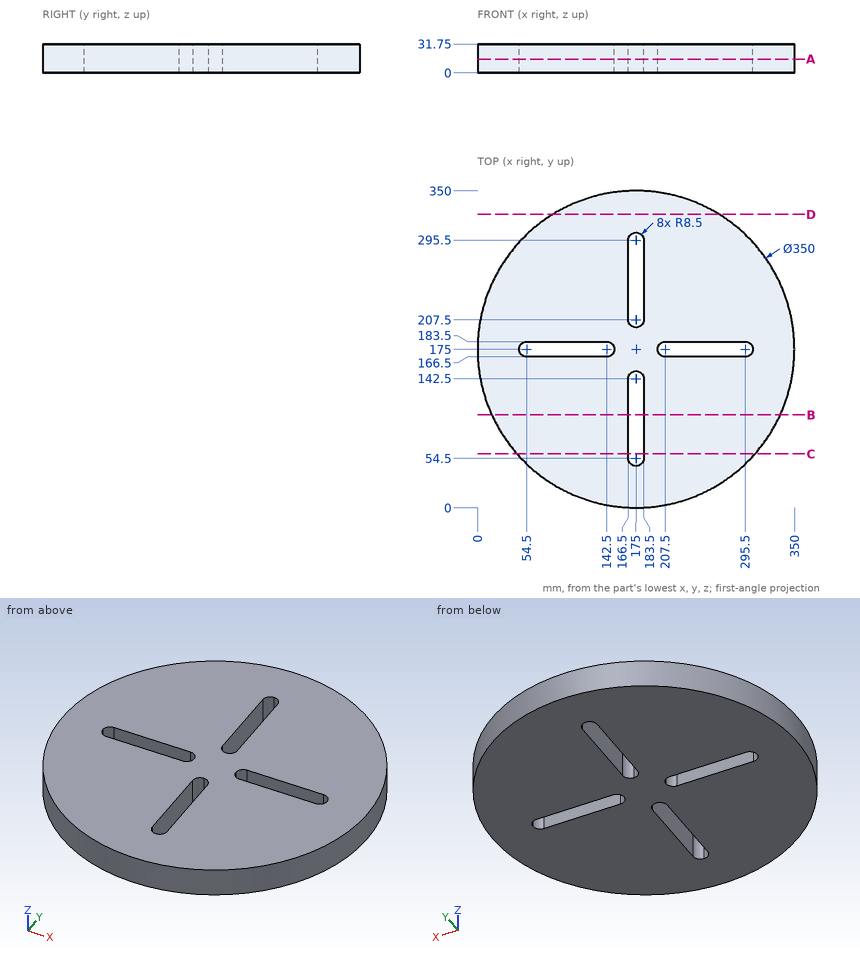
Could you check a few things on this drawing? It's one solid part, dimensions in mm from its lowest x, y, z. Give positions to 0.01 mm unless a question says otherwise; leave off trailing zeros. Write each loop counter-clockwise with the first axis right and the second up, starting at its lowest first coordinate (ties: lowest second). Pieces come first, ordered by that corner, then holes. Notation, with made-up numbers: (-36, 72.5) -> (0, 72.5) arc R17 cw to (0, 93.5) -> close; hole circle Ø10 at (84, 12.5). An arc over 180 degrees is marked (long way). Answer as CSV lines item,"result". Start each with the question number.
(1) If we section it at A-A, the plane z = 15: Write out the boundary of the cut face in (x, y).
(2) If we section it at C-C, the plane y = 59.5: Write out the boundary of the cut face in (x, z), and give its area (3 significant figures).
(3) I'm going to push flat-ended pins straight in: pin 1 Ø16 at (x, z) = (266, 20.5) entering from +Y; pin 2 Ø8 at (x, z) = (111, 18.5) entering from +Y; pin 3 Ø9.5 at (x, z) = (102, 13.5) entering from -Y. Where does each tip first touch, or does it pass through?
(4) If we section it at B-B, the plane y = 102.5: Write out the boundary of the cut face in (x, z).
(5) If we section it at D-D, the plane y = 324: Write out the boundary of the cut face in (x, z).
(6) Please list where these lines run through material, in increasing order: line 1 (Y direction, x = 127.5, z = 2); line 2 (X direction, y = 287, z = 22.5); line 3 (Y direction, x = 291, z = 3.5).
Answer list:
1,outline,"circle Ø350 at (175, 175); hole (46, 175) arc R8.5 ccw to (54.5, 166.5) -> (142.5, 166.5) arc R8.5 ccw to (151, 175) arc R8.5 ccw to (142.5, 183.5) -> (54.5, 183.5) arc R8.5 ccw to start; hole (166.5, 54.5) arc R8.5 ccw to (175, 46) arc R8.5 ccw to (183.5, 54.5) -> (183.5, 142.5) arc R8.5 ccw to (175, 151) arc R8.5 ccw to (166.5, 142.5) -> close; hole (166.5, 207.5) arc R8.5 ccw to (175, 199) arc R8.5 ccw to (183.5, 207.5) -> (183.5, 295.5) arc R8.5 ccw to (175, 304) arc R8.5 ccw to (166.5, 295.5) -> close; hole (199, 175) arc R8.5 ccw to (207.5, 166.5) -> (295.5, 166.5) arc R8.5 ccw to (304, 175) arc R8.5 ccw to (295.5, 183.5) -> (207.5, 183.5) arc R8.5 ccw to start"
2,outline,"(43.53, 0) -> (166.5, 0) -> (166.5, 31.75) -> (43.53, 31.75) -> close; (183.5, 0) -> (306.47, 0) -> (306.47, 31.75) -> (183.5, 31.75) -> close"
2,area,"7,810 mm^2"
3,pin 1,"y = 329.06"
3,pin 2,"y = 339.39"
3,pin 3,"y = 13.86"
4,outline,"(15.72, 0) -> (166.5, 0) -> (166.5, 31.75) -> (15.72, 31.75) -> close; (183.5, 0) -> (334.28, 0) -> (334.28, 31.75) -> (183.5, 31.75) -> close"
5,outline,"(83.22, 0) -> (266.78, 0) -> (266.78, 31.75) -> (83.22, 31.75) -> close"
6,line 1,"6.57 to 166.5, 183.5 to 343.43"
6,line 2,"40.53 to 166.5, 183.5 to 309.47"
6,line 3,"43.97 to 166.5, 183.5 to 306.03"
